Design review of the part built by this model. Coordinates are the model's own, in mm. A direction names the side the tool comes from. Coordinates: 2 decimals unless noted, no trailing zeros. Write each loop counter-clockwise with the first axis right and the second up, starting at its lowest first coordinate (ties: lowest second). Pieces come first, ordered by that corner, then holes.
Q1. Machinability: for faces 1 (the flat face through (28.75, 0, 26)), 2 (the flat face through (35, -1, 50)), 3 (the flat face through (-0.2, 4.25, 2.7)), 4 (the flat face through (-31.75, 0, 23)), 5 (the flat face through (33, 0, 47)), which of the approach directions +Z, -Z, +X, -X, +Y, -Y give a long, thin tool a straight path to every point of the face, cutting with its end or side? Answer none if there is none.
Q2. Take a section at B-B (x = -25.4). Give the boundary of the cut face in (y, z).
Q3. Take a section at A-A (z = 13). Give the boundary of the cut face in (x, y), and give its area (3 significant figures).
Q4. Take a section at D-D (x = 36.75). Give the boundary of the cut face in (y, z).
Q5. Take a section at C-C (y = 0). State how many separate pieces and enclosed holes the cut face has, and give its area (3 significant figures).
Q6. Mouldability with a two-part tool opening along Y and no side actions: class faces 6 (the flat face through (-33, 0, 47)), 7 (the flat face through (-0.2, -4.25, 2.7)), 8 (the cylindrical face through (38.1, 1.03, 49.34)), 9 (the cylindrical face through (-40.998, 3.537, 48.521)) as pulls with the +Y half, pulls with the -Y half, needs draft (parallel to the pull), parting line crosses it, or undercut.
Q7. Insertion check: pin 1 (2.5 mm diameter, centred on x = -8, y = 0.5, fed in from +Z); pin 2 (4 mm diameter, centred on x = -35, y = -1, fed in from -Z); pin 3 (2.5 mm diameter, centred on y = 0.5, z = 17, fed in from -X). Each pin has a flat end and moves straight along its axis. Give the tip position at first contact, or say it passes through.
Q8. For probe 1 along Y at (x, z) = (25.4, 1.85); probe 2 along Y at (x, z) = (36.75, 48.95); probe 3 along X at (y, z) = (-3.5, 23.5), list the stretches that pass through material, from the lowest coordinate up.
```python
from build123d import *

# Parameters (mm, degrees)
F0_W            = 63.5
F0_H            = 8.5
F0_R            = 1.25
F1_DEPTH        = 3
F2_W            = 3
F2_H            = 8.5
F3_DEPTH        = 47
F4_W            = 8.5
F4_H            = 3
F5_DEPTH        = 10
F6_W            = 8.5
F6_H            = 3
F7_DEPTH        = 10
F9_D            = 3.4
F9_DEPTH        = 5
F9_CSINK_D      = 6.72
F9_CSINK_ANGLE  = 90
F9_TIP          = 1.0214630523
F11_D           = 3.4
F11_DEPTH       = 5
F11_CSINK_D     = 6.72
F11_CSINK_ANGLE = 90
F11_TIP         = 1.0214630523
F12_R           = 2.5


with BuildPart() as f1:
    # F0 (on Top) → F1 (new body)
    with BuildSketch(Plane.XY):
        Rectangle(F0_W, F0_H)
        with Locations((-25.4, 0)):
            Circle(F0_R, mode=Mode.SUBTRACT)
        with Locations((25.4, 0)):
            Circle(F0_R, mode=Mode.SUBTRACT)
    extrude(amount=F1_DEPTH)

    # F2 (on face) → F3 (join)
    with BuildSketch(Plane.XY.offset(3)):
        with Locations((-30.25, 0)):
            Rectangle(F2_W, F2_H)
        with Locations((30.25, 0)):
            Rectangle(F2_W, F2_H)
    extrude(amount=F3_DEPTH)

    # F4 (on face) → F5 (join)
    with BuildSketch(Plane(origin=(-31.75, 0, 0), x_dir=(0, -1, 0), z_dir=(-1, 0, 0))):
        with Locations((0, 48.5)):
            Rectangle(F4_W, F4_H)
    extrude(amount=F5_DEPTH)

    # F6 (on face) → F7 (join)
    with BuildSketch(Plane.YZ.offset(31.75)):
        with Locations((0, 48.5)):
            Rectangle(F6_W, F6_H)
    extrude(amount=F7_DEPTH)

    # F9
    with Locations(Plane(origin=(0, 0, 47), x_dir=(1, 0, 0), z_dir=(0, 0, -1))):
        with Locations((-36.75, 0)):
            CounterSinkHole(F9_D / 2, F9_CSINK_D / 2, depth=F9_DEPTH, counter_sink_angle=F9_CSINK_ANGLE)
            with Locations((0, 0, -(F9_DEPTH + F9_TIP / 2))):  # 118° drill point
                Cone(0, F9_D / 2, F9_TIP, mode=Mode.SUBTRACT)

    # F11
    with Locations(Plane(origin=(0, 0, 47), x_dir=(1, 0, 0), z_dir=(0, 0, -1))):
        with Locations((36.75, 0)):
            CounterSinkHole(F11_D / 2, F11_CSINK_D / 2, depth=F11_DEPTH, counter_sink_angle=F11_CSINK_ANGLE)
            with Locations((0, 0, -(F11_DEPTH + F11_TIP / 2))):  # 118° drill point
                Cone(0, F11_D / 2, F11_TIP, mode=Mode.SUBTRACT)

    # F12
    f12_edges = [f1.edges().sort_by_distance(p)[0] for p in [
        (41.75, 4.25, 48.5),
        (41.75, -4.25, 48.5),
        (-41.75, 4.25, 48.5),
        (-41.75, -4.25, 48.5),
    ]]
    fillet(f12_edges, radius=F12_R)


solid = f1.part
```
Response:
1. face 1: +Z, +Y, -Y
1. face 2: +Z, +X, -X, +Y, -Y
1. face 3: +Z, -Z, +X, -X, +Y
1. face 4: -Z, -X, +Y, -Y
1. face 5: -Z, +X, +Y, -Y
2. outline: (-4.25, 0) - (-1.25, 0) - (-1.25, 3) - (-4.25, 3) - close; (1.25, 0) - (4.25, 0) - (4.25, 3) - (1.25, 3) - close
3. outline: (-31.75, -4.25) - (-28.75, -4.25) - (-28.75, 4.25) - (-31.75, 4.25) - close; (28.75, -4.25) - (31.75, -4.25) - (31.75, 4.25) - (28.75, 4.25) - close
3. area: 51.0 mm2
4. outline: (-4.25, 47) - (-3.36, 47) - (-1.7, 48.66) - (-1.7, 50) - (-4.25, 50) - close; (1.7, 48.66) - (3.36, 47) - (4.25, 47) - (4.25, 50) - (1.7, 50) - close
5. separate pieces: 5
5. enclosed holes: 0
5. area: 492 mm2
6. face 6: needs draft
6. face 7: pulls with the -Y half
6. face 8: undercut
6. face 9: pulls with the +Y half
7. pin 1: stops at z = 3
7. pin 2: stops at z = 47
7. pin 3: stops at x = -31.75
8. probe 1: y = -4.25 to -1.25, 1.25 to 4.25
8. probe 2: y = -4.25 to -1.7, 1.7 to 4.25
8. probe 3: x = -31.75 to -28.75, 28.75 to 31.75
